The figure shows three views and two pictorial views of one solid part (mm, origin at its lowest corner). Answer the questions. A direction names the side the tool comes from. Round coordinates to 2 decimals unless told otherwise and drop trailing zeros. Order: outer loops, then holes, each group sorted by start corner. A loop starts at its lowest first (then second) coordinate and runs counter-clockwise, first axis right, second up. Notation, with made-up numbers: (2.25, -20) - (12.25, -20) arc R22 cw to (12.25, -13) - close; hole circle Ø11 at (26.5, 15.25). An arc over 180 degrees is marked (long way). Answer in a Markdown table with one row per item.
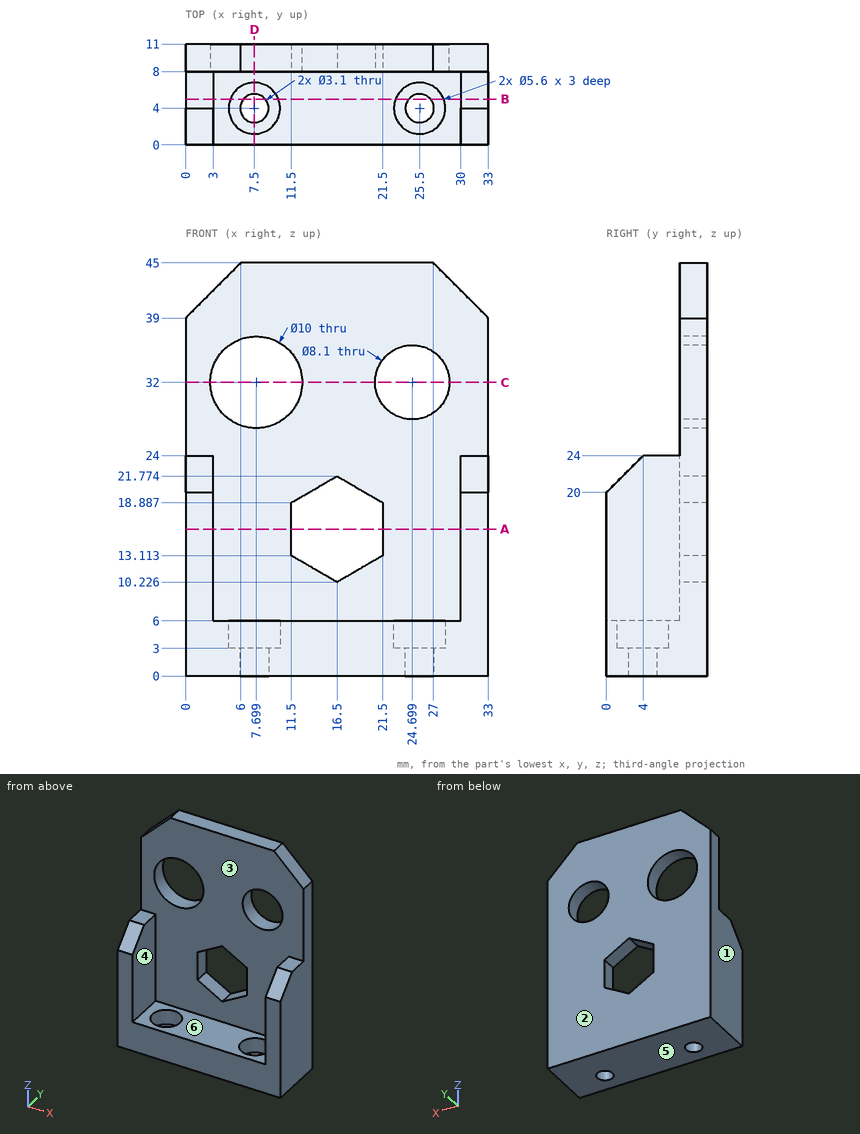
1) Find section B-B, the plane y = 5. Give the vertices of the cut face in (x, z) (1 decimal).
Filled in:
| item | result |
|---|---|
| outline | (0, 0) - (6.3, 0) - (6.3, 3) - (4.9, 3) - (4.9, 6) - (3, 6) - (3, 24) - (0, 24) - close; (8.7, 0) - (24.3, 0) - (24.3, 3) - (22.9, 3) - (22.9, 6) - (10.1, 6) - (10.1, 3) - (8.7, 3) - close; (26.7, 0) - (33, 0) - (33, 24) - (30, 24) - (30, 6) - (28.1, 6) - (28.1, 3) - (26.7, 3) - close |
2) Which of the six approach directions +Z, -Z, +X, -X, +Y, -Y give full straight-line access (tool end or side, diameter ignored) to the marked faces 5 and 6?
Filled in:
| item | result |
|---|---|
| face 5 | -Z, +X, -X, +Y, -Y |
| face 6 | +Z, -Y |
3) Each of these flat-tipped pins is pushed along its axis until it touches: pin 1 (3.5 mm diameter, centred on x = 1, y = 5.5, fed in from +Z); pin 2 (8 mm diameter, centred on x = 25, z = 29, fed in from -Y); pin 3 (4 mm diameter, centred on x = 7.5, y = 4, fed in from +Z). Where does it stop, or does it pass through?
Filled in:
| item | result |
|---|---|
| pin 1 | stops at z = 24 |
| pin 2 | stops at y = 8 |
| pin 3 | stops at z = 3 |
4) Find section C-C, the plane z = 32. Give the vertices of the cut face in (x, y).
Filled in:
| item | result |
|---|---|
| outline | (0, 8) - (2.7, 8) - (2.7, 11) - (0, 11) - close; (12.7, 8) - (20.65, 8) - (20.65, 11) - (12.7, 11) - close; (28.75, 8) - (33, 8) - (33, 11) - (28.75, 11) - close |
5) Find the intervals of material crossed by probe 1 along Z at (x, y) = (7.5, 8.25) (1 decimal); probe 2 along X at (y, z) = (9.3, 32); probe 3 along X at (y, z) = (9.5, 33.5), in increasing order. Write a range as from..to.
Filled in:
| item | result |
|---|---|
| probe 1 | z = 0..27, 37..45 |
| probe 2 | x = 0..2.7, 12.7..20.65, 28.75..33 |
| probe 3 | x = 0..2.93, 12.47..20.94, 28.46..33 |
6) Find section D-D, the plane x = 7.5. Give the vertices of the cut face in (y, z).
Filled in:
| item | result |
|---|---|
| outline | (0, 0) - (2.45, 0) - (2.45, 3) - (1.2, 3) - (1.2, 6) - (0, 6) - close; (5.55, 0) - (11, 0) - (11, 27) - (8, 27) - (8, 6) - (6.8, 6) - (6.8, 3) - (5.55, 3) - close; (8, 37) - (11, 37) - (11, 45) - (8, 45) - close |
7) The mould has two halves that part along X. Classify the marked faces 1, 2, 3 and 4: released by +X, released by -X, zero draft, split by the parting line, or undercut.
Filled in:
| item | result |
|---|---|
| face 1 | released by -X |
| face 2 | zero draft |
| face 3 | undercut |
| face 4 | undercut |
8) Find section A-A, the plane z = 16. Give the vertices of the cut face in (x, y).
Filled in:
| item | result |
|---|---|
| outline | (0, 0) - (3, 0) - (3, 8) - (11.5, 8) - (11.5, 11) - (0, 11) - close; (21.5, 8) - (30, 8) - (30, 0) - (33, 0) - (33, 11) - (21.5, 11) - close |
